Geometry check sheet. Reference: drawing and pictorial views, mm from the part's lowest x, y, z. A direction names the side the tool comes from. Coordinates: 2 decimals unless noted, no trailing zeros. Write each loop counter-clockwise with the first axis right and the second up, starting at its lowest first coordinate (ties: lowest second). Pieces come first, ordered by that corner, then holes. Notation, with made-up numbers: M -22.5,66.5 L 34.5,66.5 A35 ccw 34.5,103.5 Z; hole C 6.25,6.25 d5. An arc over 180 degrees is marked long. One line per item, written item: value.
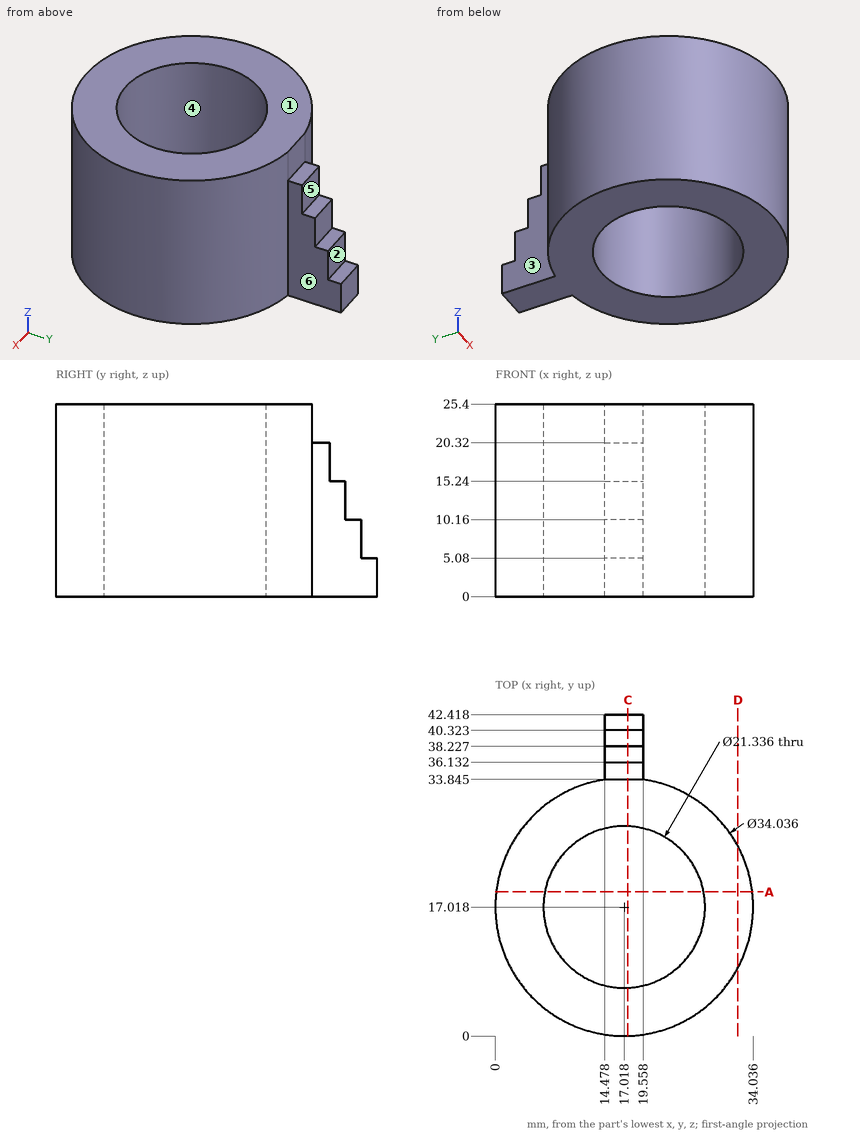
Item 1: Cross-section at D-D, the plane x = 32. Enter the section's corners in (y, z).
The answers:
outline: M 8.95,0 L 25.09,0 L 25.09,25.4 L 8.95,25.4 Z
Item 2: Access from +Z, -Z, +X, -X, +Y, -Y to the whole of each face (thin tool, end or side, straight path). Record for the marked faces 1, 2 and 3.
The answers:
face 1: +Z, +X, -X, +Y, -Y
face 2: +Z, +X, -X, +Y
face 3: +Z, -Z, -X, +Y
Item 3: Scan lines: line 1 (X direction, y = 34, z = 18.25); line 2 (Y direction, x = 9, z = 9.5) (1 decimal); line 3 (Y direction, x = 11, z = 11) (1 decimal). Record each from-to range of solid material in increasing order.
The answers:
line 1: x = 14.48 to 19.56
line 2: y = 2 to 10, 24.1 to 32
line 3: y = 1.1 to 8.2, 25.8 to 32.9
Item 4: Cross-section at C-C, the plane x = 17.5. Enter the section's corners in (y, z) (1 decimal).
The answers:
outline: M 0,0 L 6.4,0 L 6.4,25.4 L 0,25.4 Z; M 27.7,0 L 42.4,0 L 42.4,5.1 L 40.3,5.1 L 40.3,10.2 L 38.2,10.2 L 38.2,15.2 L 36.1,15.2 L 36.1,20.3 L 33.8,20.3 L 33.8,25.4 L 27.7,25.4 Z
Item 5: Draft check along Y on the marked faces 4, 5 and 6. Enter one of: released by +Y, released by -Y, zero draft, split by the parting line, or undercut.
The answers:
face 4: undercut
face 5: released by +Y
face 6: zero draft
Item 6: Go/stop test with flat-tipped pins: P1, Ø12, axis at y = 27.5, z = 3, coming from the -X side; P2, Ø2.5, axis at x = 17.5, z = 7, coming from the +Y side; P3, Ø5.5, axis at x = 18, z = 24, coming from the +Y side (1 decimal). Record where each tip stops, or that it passes through.
The answers:
P1: stops at x = 0.6
P2: stops at y = 40.32
P3: stops at y = 33.8
Item 7: Cross-section at A-A, the plane y = 19. Enter the section's corners in (x, z) (1 decimal).
The answers:
outline: M 0.1,0 L 6.5,0 L 6.5,25.4 L 0.1,25.4 Z; M 27.5,0 L 33.9,0 L 33.9,25.4 L 27.5,25.4 Z
